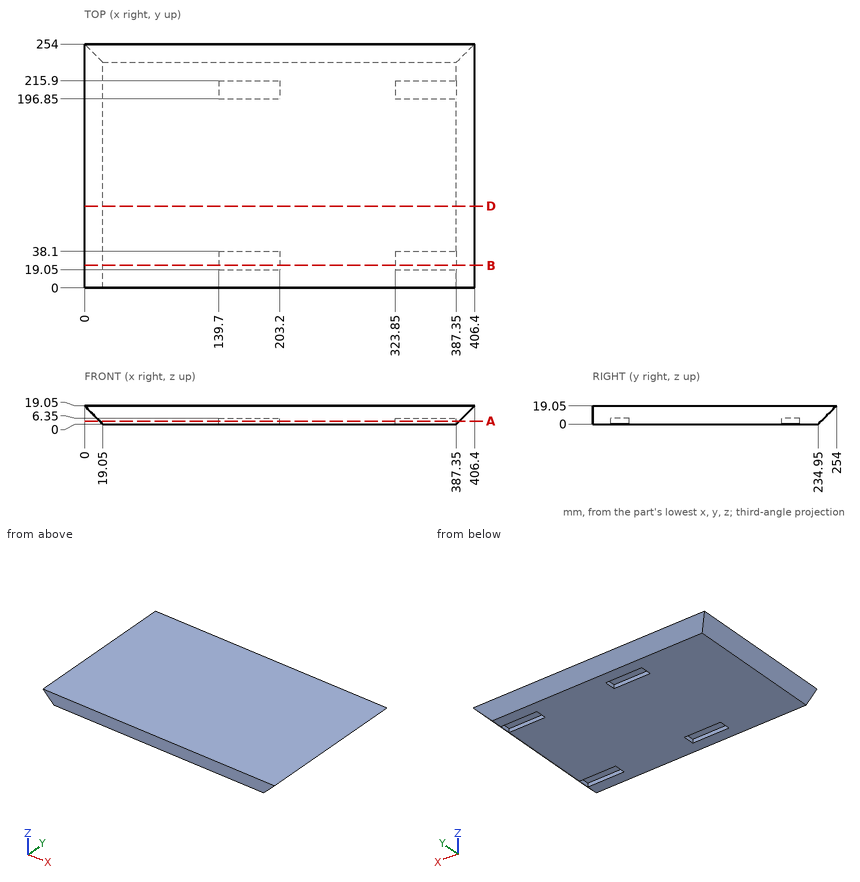
Study the drawing (mm; zero at the part's minimum x, y, z) and answer. Coordinates: 2 decimals unless noted, no trailing zeros. Order: outer loops, then holes, each group sorted by start corner. A loop starts at its lowest first (then second) coordinate and runs counter-clockwise, first axis right, second up. Notation, with made-up numbers: (32.25, 44.25) -> (82.25, 44.25) arc R29 cw to (82.25, 76.25) -> close; hole circle Ø5 at (-3.5, 55.5). An arc over 180 degrees is marked (long way). Answer in a Markdown table with one row per item. Add a question column.
Item 1: Find section D-D (y = 85). Write down the section's boundary in (x, z), then the cut area to 3 significant figures.
Item 2: Each of these flat-tipped pins is pushed along its axis until it touches: P1, Ø7, axis at y = 32.5, z = 3, coming from the -X side; P2, Ø1.5, axis at x = 218.5, z = 11, coming from the +Y side; P3, Ø1.9, axis at y = 30, z = 3.5, coming from the -X side. Where does it stop, or does it pass through?
Item 3: Find the intervals of material crossed by L1, parallel to Y at x = 186.5, z = 4.75; L2, parallel to Y at x = 167.5, z = 4.5; L3, parallel to X at y = 208, z = 5.75, in increasing order. Write a range as from..to.
Item 4: Find section A-A (z = 3.25). Write down the section's boundary in (x, y), then the cut area to 3 significant figures.
Item 5: Find section B-B (y = 23.5). Write down the section's boundary in (x, z).
Result set:
| question | item | result |
|---|---|---|
| 1 | outline | (0, 19.05) -> (19.05, 0) -> (387.35, 0) -> (406.4, 19.05) -> close |
| 1 | area | 7,380 mm² |
| 2 | P1 | stops at x = 12.55 |
| 2 | P2 | stops at y = 246.7 |
| 2 | P3 | stops at x = 14.6 |
| 3 | L1 | y = 0..19.05, 38.1..196.85, 215.9..239.7 |
| 3 | L2 | y = 0..19.05, 38.1..196.85, 215.9..239.45 |
| 3 | L3 | x = 13.3..139.7, 203.2..323.85, 387.35..393.1 |
| 4 | outline | (15.8, 0) -> (390.6, 0) -> (390.6, 238.2) -> (15.8, 238.2) -> close; hole (139.7, 19.05) -> (203.2, 19.05) -> (203.2, 38.1) -> (139.7, 38.1) -> close; hole (139.7, 196.85) -> (203.2, 196.85) -> (203.2, 215.9) -> (139.7, 215.9) -> close; hole (323.85, 19.05) -> (387.35, 19.05) -> (387.35, 38.1) -> (323.85, 38.1) -> close; hole (323.85, 196.85) -> (387.35, 196.85) -> (387.35, 215.9) -> (323.85, 215.9) -> close |
| 4 | area | 84,400 mm² |
| 5 | outline | (0, 19.05) -> (19.05, 0) -> (139.7, 0) -> (139.7, 6.35) -> (203.2, 6.35) -> (203.2, 0) -> (323.85, 0) -> (323.85, 6.35) -> (387.35, 6.35) -> (387.35, 0) -> (406.4, 19.05) -> close |
